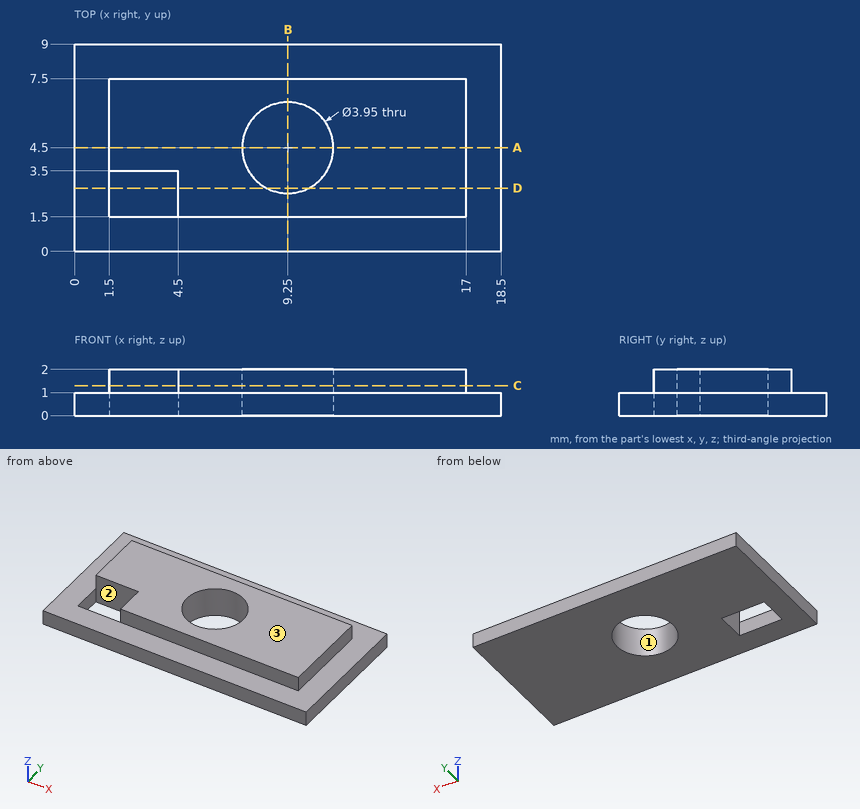
Answer from the drawing. Dimensions are ordinates in mm from the lowest x, y and z of the part. Round coordinates to 2 decimals unless told otherwise and drop trailing zeros. Loops run counter-clockwise (first coordinate to the right, second up) from the corner with the lowest first, then second, coordinate; pieces in that order, holes last.
Q1. Determine the mould class of the marked faces 1, 2 and 3 for opening direction X: released by +X, released by -X, zero draft, split by the parting line, or undercut.
Q2. Consider probe 1 along Y at (x, z) = (4, 0.85); probe 2 along Y at (x, z) = (9.25, 1.3) (3 decimals); probe 3 along X at (y, z) = (4.75, 0.4). Determine where each line is inside the solid, lowest interval first.
Q3. Section D-D on y = 2.75 is taken. Write down the section's boundary in (x, z), and give its area (3 significant figures).
Q4. Section A-A on y = 4.5 is taken. Write down the section's boundary in (x, z) (3 decimals), and give its area (3 significant figures).
Q5. Section B-B on x = 9.25 is taken. Write down the section's boundary in (y, z) (3 decimals), and give its area (3 significant figures).
Q6. Section C-C on z = 1.3 is taken. Write down the section's boundary in (x, y) (3 decimals), and give its area (3 significant figures).
Q7. Each of these flat-tipped pins is pushed along its axis until it touches: pin 1 (0.8 mm diameter, centred on x = 9, z = 1.5, fed in from +Y); pin 2 (0.5 mm diameter, centred on y = 5, z = 1.5, fed in from -X). Where does it stop, or does it pass through?
Output:
1. face 1: undercut
1. face 2: undercut
1. face 3: zero draft
2. probe 1: y = 0 to 1.5, 3.5 to 9
2. probe 2: y = 1.5 to 2.525, 6.475 to 7.5
2. probe 3: x = 0 to 7.29, 11.21 to 18.5
3. outline: (0, 0) - (1.5, 0) - (1.5, 1) - (0, 1) - close; (4.5, 0) - (8.33, 0) - (8.33, 2) - (4.5, 2) - close; (10.17, 0) - (18.5, 0) - (18.5, 1) - (17, 1) - (17, 2) - (10.17, 2) - close
3. area: 24.3 mm2
4. outline: (0, 0) - (7.275, 0) - (7.275, 2) - (1.5, 2) - (1.5, 1) - (0, 1) - close; (11.225, 0) - (18.5, 0) - (18.5, 1) - (17, 1) - (17, 2) - (11.225, 2) - close
4. area: 26.1 mm2
5. outline: (0, 0) - (2.525, 0) - (2.525, 2) - (1.5, 2) - (1.5, 1) - (0, 1) - close; (6.475, 0) - (9, 0) - (9, 1) - (7.5, 1) - (7.5, 2) - (6.475, 2) - close
5. area: 7.10 mm2
6. outline: (1.5, 3.5) - (4.5, 3.5) - (4.5, 1.5) - (17, 1.5) - (17, 7.5) - (1.5, 7.5) - close; hole circle Ø3.95 at (9.25, 4.5)
6. area: 74.7 mm2
7. pin 1: stops at y = 7.5
7. pin 2: stops at x = 1.5
